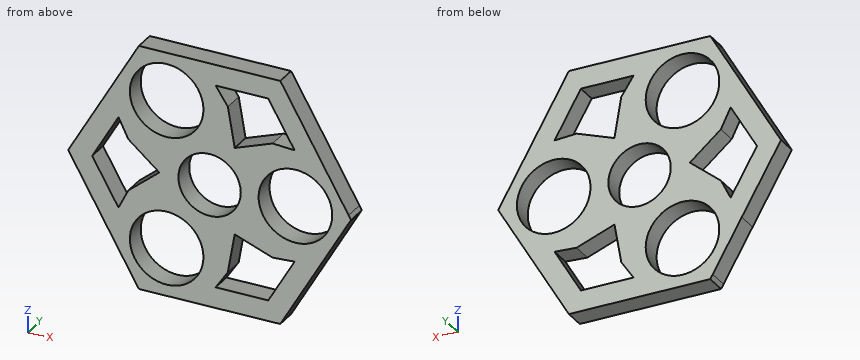
```python
from build123d import *

# Parameters (mm, degrees)
F0_R     = 11.2395
F0_R_2   = 9.525
F1_DEPTH = 6.35


# Not quite as in the source:
# - ends of sketch curves that miss each other by under 0.0002 mm in the source are joined


with BuildPart() as f1:
    # F0 (on Front) → F1 (new body)
    with BuildSketch(Plane.XZ):
        with BuildLine():
            Line((42.4467651581, 1.27), (33.5675281941, 16.6492895541))
            Line((33.5675281941, 16.6492895541), (21.59, 37.3949769354))
            Line((21.59, 37.3949769354), (-2.3645964913, 37.3949769354))
            Line((-2.3645964913, 37.3949769354), (-20.1235303163, 37.3949769354))
            ThreePointArc((-20.1235303163, 37.3949769354), (-21.3935303163, 37.054681461), (-22.3232348419, 36.1249769354))
            Line((-22.3232348419, 36.1249769354), (-31.2024718059, 20.7456873813))
            Line((-31.2024718059, 20.7456873813), (-43.18, 0))
            Line((-43.18, 0), (-31.2027017544, -20.7452890988))
            Line((-31.2027017544, -20.7452890988), (-22.3232348418, -36.1249769356))
            ThreePointArc((-22.3232348418, -36.1249769356), (-21.9195815404, -36.6510281597), (-21.3935303163, -37.0546814611))
            ThreePointArc((-21.3935303163, -37.0546814611), (-20.7809306909, -37.3084285342), (-20.1235303165, -37.3949769354))
            Line((-20.1235303165, -37.3949769354), (-2.3645964913, -37.3949769354))
            Line((-2.3645964913, -37.3949769354), (21.59, -37.3949769354))
            Line((21.59, -37.3949769354), (33.5675281941, -16.6492895541))
            Line((33.5675281941, -16.6492895541), (42.4467651581, -1.27))
            ThreePointArc((42.4467651581, -1.27), (42.7870606325, 0), (42.4467651581, 1.27))
        make_face()
        with Locations((-13.1097560234, -22.7067635073)):
            Circle(F0_R, mode=Mode.SUBTRACT)
        Polygon((1.8552556307, -31.0449769354), (5.579663063, -25.4405181745), (7.6765207659, -13.2964418818), (19.2425445444, -17.5521669359), (25.957862804, -17.1289127727), (17.9235712565, -31.0449769354), align=None, mode=Mode.SUBTRACT)
        Polygon((-15.3532430276, -9.74608e-05), (-24.8219665561, -7.8881291301), (-24.8578663434, -7.9604670809), (-27.8131295737, -13.9154964701), (-35.8475243142, 0.000220433), (-27.8133665013, 13.915789961), (-24.8219665561, 7.8881291301), align=None, mode=Mode.SUBTRACT)
        with Locations((-13.1097560234, 22.7067635073)):
            Circle(F0_R, mode=Mode.SUBTRACT)
        Circle(F0_R_2, mode=Mode.SUBTRACT)
        with Locations((26.2195120463, 0.0001612286)):
            Circle(F0_R, mode=Mode.SUBTRACT)
        Polygon((7.6765207659, 13.2964418818), (5.579663063, 25.4405181745), (1.8552556307, 31.0449769354), (17.9235712565, 31.0449769354), (25.957862804, 17.1289127727), (19.2425445444, 17.5521669359), align=None, mode=Mode.SUBTRACT)
        with BuildLine():
            Line((43.18, 0), (42.4467651581, 1.27))
            ThreePointArc((42.4467651581, 1.27), (42.7870606325, 0), (42.4467651581, -1.27))
            Line((42.4467651581, -1.27), (43.18, 0))
        make_face()
        with BuildLine():
            ThreePointArc((-22.3232348419, 36.1249769354), (-21.3935303163, 37.054681461), (-20.1235303163, 37.3949769354))
            Line((-20.1235303163, 37.3949769354), (-21.59, 37.3949769354))
            Line((-21.59, 37.3949769354), (-22.3232348419, 36.1249769354))
        make_face()
        with BuildLine():
            Line((-21.59, -37.3949769354), (-20.1235303165, -37.3949769354))
            ThreePointArc((-20.1235303165, -37.3949769354), (-20.7809306909, -37.3084285342), (-21.3935303163, -37.0546814611))
            Line((-21.3935303163, -37.0546814611), (-21.59, -37.3949769354))
        make_face()
        with BuildLine():
            Line((-21.59, -37.3949769354), (-21.3935303163, -37.0546814611))
            ThreePointArc((-21.3935303163, -37.0546814611), (-21.9195815404, -36.6510281597), (-22.3232348418, -36.1249769356))
            Line((-22.3232348418, -36.1249769356), (-21.59, -37.3949769354))
        make_face()
    extrude(amount=F1_DEPTH)


solid = f1.part
```
Could you check a few things on this model? Use its own coordinates, in mm. Give positions to 0.01 mm unless a question says otherwise; leave off trailing zeros. Write each loop counter-clockwise with the first axis right and the second up, starting at its lowest first coordinate (ties: lowest second). Pieces come first, ordered by that corner, then holes. Notation, with made-up numbers: (19, 55) - (71, 55) arc R26 ccw to (71, 71) - close; hole circle Ø7 at (66.25, 27.25). An arc over 180 degrees is marked (long way). One line per item, written item: value. Start each with the question number.
Item 1: I'm going to push a flat-ended pin straight in: pin 1 (2 mm diameter, centred on x = 27.5, y = -5.5, fed in from -Z). Where does the tip first touch, or does it pass through?
Item 2: Imagine slicing it at D-D, the plane x = 29.5. List the corners of the cut face in (y, z) for me.
Item 3: Imagine slicing it at B-B, the plane z = -4.5. List the corners of the cut face in (x, y) for me, and give its area (3 significant figures).
Item 4: Imagine slicing it at A-A, the plane x = 0. List the corners of the cut face in (y, z) for me (3 decimals), and give its area (3 significant figures).
Item 5: Imagine slicing it at C-C, the plane y = -2.75. Give the number of separate pieces and of enclosed holes in the cut face, and give its area (3 significant figures).
Item 6: Please list where these lines run through material, in increasing order: line 1 (Z direction, x = -12.5, y = -2); line 2 (Z direction, x = 0, y = -3.5) (3 decimals); line 3 (Z direction, x = 22.5, y = -3). Write a range as from..to.
Geometry says:
1. pin 1: z = -28.89
2. outline: (-6.35, -23.69) - (0, -23.69) - (0, -10.75) - (-6.35, -10.75) - close; (-6.35, 10.75) - (0, 10.75) - (0, 23.69) - (-6.35, 23.69) - close
3. outline: (-40.58, -6.35) - (-33.25, -6.35) - (-33.25, 0) - (-40.58, 0) - close; (-20.75, -6.35) - (-8.39, -6.35) - (-8.39, 0) - (-20.75, 0) - close; (8.39, -6.35) - (15.92, -6.35) - (15.92, 0) - (8.39, 0) - close; (36.52, -6.35) - (40.58, -6.35) - (40.58, 0) - (36.52, 0) - close
3. area: 199 mm^2
4. outline: (-6.35, -37.395) - (0, -37.395) - (0, -9.525) - (-6.35, -9.525) - close; (-6.35, 9.525) - (0, 9.525) - (0, 37.395) - (-6.35, 37.395) - close
4. area: 354 mm^2
5. separate pieces: 1
5. enclosed holes: 7
5. area: 2,610 mm^2
6. line 1: -37.39..-33.93, -11.48..11.48, 33.93..37.39
6. line 2: -37.395..-9.525, 9.525..37.395
6. line 3: -35.82..-23.12, -17.35..-10.61, 10.61..17.35, 23.12..35.82
